Work out the finished part from the listing and answer in its coordinate system (mm). A direction names the side the tool comes from. Round coordinates to 2 decimals unless told otherwise and drop trailing zeros. Order: outer loops, then holes, each group sorted by start corner. A loop starts at its lowest first (then second) coordinate and runs counter-clockwise, first axis right, second up. Notation, with made-up numbers: M 39.5,2.25 L 94.5,2.25 A8 ccw 94.5,7.25 Z; hole C -4,36 d10. An arc over 180 degrees is marked long. Return JSON: item names as keys, results as strings.
from build123d import *

# Parameters (mm, degrees)
F1_DEPTH = 41.91
F3_DEPTH = 52.832
F4_R     = 10.605474
F5_DEPTH = 85.598
F6_W     = 33.727639
F6_H     = 19.182933
F7_DEPTH = 56.896


with BuildPart() as f1:
    # F0 (on Top) → F1 (new body)
    with BuildSketch(Plane.XY):
        with BuildLine():
            Line((0, 101.6), (0, -101.6))
            Line((0, -101.6), (152.4, -101.6))
            ThreePointArc((152.4, -101.6), (188.321024, -86.721024), (203.2, -50.8))
            Line((203.2, -50.8), (101.6, -50.8))
            Line((101.6, -50.8), (101.6, 50.8))
            Line((101.6, 50.8), (203.2, 50.8))
            ThreePointArc((203.2, 50.8), (188.321024, 86.721024), (152.4, 101.6))
            Line((152.4, 101.6), (0, 101.6))
        make_face()
    extrude(amount=F1_DEPTH)

    # F2 (on face) → F3 (join)
    with BuildSketch(Plane(origin=(0, 0, 0), x_dir=(0, -1, 0), z_dir=(-1, 0, 0))):
        Polygon((-27.380493, 93.494549), (-101.6, 41.91), (101.6, 41.91), (50.246455, 93.494549), align=None)
    extrude(amount=-F3_DEPTH)

    # F4 (on face) → F5 (cut)
    with BuildSketch(Plane.YZ.offset(52.832)):
        with Locations((-6.630837, 68.815641)):
            Circle(F4_R)
    extrude(amount=-F5_DEPTH, mode=Mode.SUBTRACT)

    # F6 (on face) → F7 (cut)
    with BuildSketch(Plane.YZ.offset(101.6)):
        with Locations((13.456206, 9.591466)):
            Rectangle(F6_W, F6_H)
    extrude(amount=-F7_DEPTH, mode=Mode.SUBTRACT)


solid = f1.part
Item 1: Which of the six approach directions +Z, -Z, +X, -X, +Y, -Y give full straight-line access (tool end or side, diameter ignored) to faces 4 (the flat face through (52.832, 1, 57)), 5 (the flat face through (152, 50.8, 21)), 6 (the flat face through (77, 101.6, 21)), 7 (the flat face through (74, 30.32, 9))?
Output:
{"face 4": "+Z, +X, +Y, -Y", "face 5": "+Z, -Z, +X", "face 6": "+Z, -Z, +X, -X, +Y", "face 7": "-Z, +X"}
Item 2: Find section C-C (y = 21). Determine the outline of the cut face in (x, z).
Output:
{"outline": "M 0,0 L 44.7,0 L 44.7,19.18 L 101.6,19.18 L 101.6,41.91 L 52.83,41.91 L 52.83,93.49 L 0,93.49 Z"}
Item 3: Find section B-B (z = 28.5). Determine the outline of the cut face in (x, y).
Output:
{"outline": "M 0,-101.6 L 152.4,-101.6 A50.8 ccw 203.2,-50.8 L 101.6,-50.8 L 101.6,50.8 L 203.2,50.8 A50.8 ccw 152.4,101.6 L 0,101.6 Z"}
Item 4: Find section A-A (x = 136). Determine the outline of the cut face in (y, z), plus the area to 3 significant figures.
Output:
{"outline": "M -101.6,0 L -50.8,0 L -50.8,41.91 L -101.6,41.91 Z; M 50.8,0 L 101.6,0 L 101.6,41.91 L 50.8,41.91 Z", "area": "4,260 mm^2"}
Item 5: Consider line 1 along Y through (x, z) = (108.5, 37); line 2 along Z through (x, y) = (54, 24.5); line 3 along Z through (x, y) = (62, -80). Determine where each line is inside the solid, lowest interval first. Write a range as [from, to].
Output:
{"line 1": "y = [-101.6, -50.8], [50.8, 101.6]", "line 2": "z = [19.18, 41.91]", "line 3": "z = [0, 41.91]"}
Item 6: Each of these flat-tipped pins is pushed along its axis until it touches: pin 1 (21 mm diameter, centred on y = 17, z = 11, fed in from +X); pin 2 (1.5 mm diameter, centred on x = 36.5, z = 82.5, fed in from +Y); pin 3 (8 mm diameter, centred on x = 174.5, z = 30.5, fed in from -Y). Where does it stop, or does it pass through?
Output:
{"pin 1": "stops at x = 101.6", "pin 2": "stops at y = 44.28", "pin 3": "stops at y = -98.27"}
Item 7: Find section D-D (z = 65.5). Determine the outline of the cut face in (x, y).
Output:
{"outline": "M 0,-78.12 L 52.83,-78.12 L 52.83,-16.7 L 0,-16.7 Z; M 0,3.44 L 52.83,3.44 L 52.83,67.66 L 0,67.66 Z"}
Item 8: The mould has two halves that part along Y. Classify faces 1 (the flat face through (101.6, -1, 21)), 2 (the flat face through (78, -21, 0)), 3 (the flat face through (26.046, -76.283, 67.341)): pulls with the +Y half, pulls with the -Y half, needs draft (parallel to the pull), parting line crosses it, or undercut.
Output:
{"face 1": "undercut", "face 2": "needs draft", "face 3": "pulls with the -Y half"}
